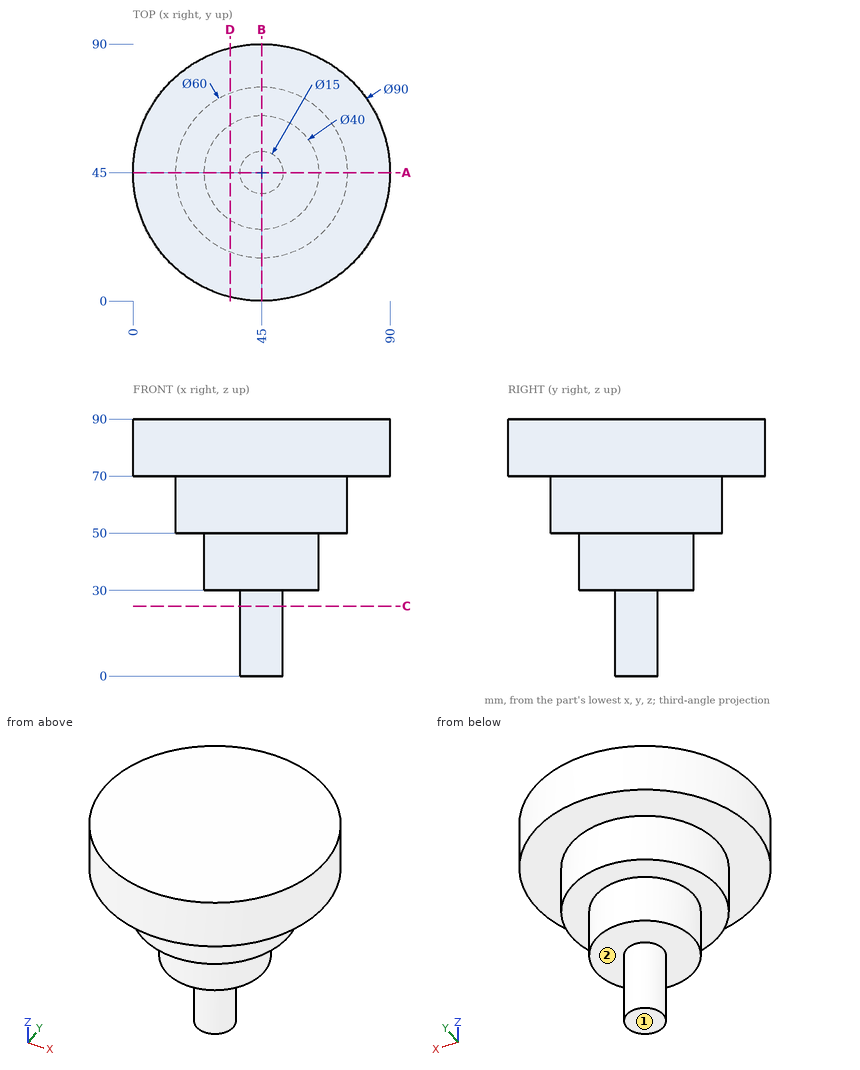
Can you work these out from the drawing? Everything is in mm from the part's minimum corner. A direction names the side the tool comes from. Round coordinates to 2 decimals unless told otherwise and drop trailing zeros. Loops run counter-clockwise (first coordinate to the right, second up) from the corner with the lowest first, then second, coordinate; pieces in that order, holes last. Notation, with made-up numbers: (-22, 10) -> (-4, 10) arc R23 cw to (-4, 23) -> close; hole circle Ø5 at (50.25, 34). An arc over 180 degrees is marked (long way). Answer in a Markdown table with one row per item.
Item 1: Suppose I cut it at D-D, the plane x = 34. List the corners of the cut face in (y, z) for me, plus the area to 3 significant figures.
Answer block:
| item | result |
|---|---|
| outline | (1.37, 70) -> (17.09, 70) -> (17.09, 50) -> (28.3, 50) -> (28.3, 30) -> (61.7, 30) -> (61.7, 50) -> (72.91, 50) -> (72.91, 70) -> (88.63, 70) -> (88.63, 90) -> (1.37, 90) -> close |
| area | 3,530 mm² |
Item 2: Suppose I cut it at A-A, the plane y = 45. List the corners of the cut face in (x, z) for me.
Answer block:
| item | result |
|---|---|
| outline | (0, 70) -> (15, 70) -> (15, 50) -> (25, 50) -> (25, 30) -> (37.5, 30) -> (37.5, 0) -> (52.5, 0) -> (52.5, 30) -> (65, 30) -> (65, 50) -> (75, 50) -> (75, 70) -> (90, 70) -> (90, 90) -> (0, 90) -> close |
Item 3: Suppose I cut it at C-C, the plane z = 24.5. List the corners of the cut face in (x, y) for me.
Answer block:
| item | result |
|---|---|
| outline | circle Ø15 at (45, 45) |
Item 4: If I drill on probe 1 along Z at (x, y) = (32, 46.5); probe 2 along X at (y, z) = (46.5, 85) (3 decimals); probe 3 along X at (y, z) = (45, 69), over which ranges is the centre line in solid material (lowest first)?
Answer block:
| item | result |
|---|---|
| probe 1 | 30 to 90 |
| probe 2 | 0.025 to 89.975 |
| probe 3 | 15 to 75 |
Item 5: Will these pins go through, and if not, where does the flat tip stop? P1, Ø3, axis at x = 41, z = 66, coming from the +Y side; P2, Ø12, axis at y = 29, z = 54, coming from the +X side; P3, Ø1.5, axis at y = 76.5, z = 57, coming from the -X side; P4, Ø1, axis at x = 17, y = 45.5, coming from the -Z side.
Answer block:
| item | result |
|---|---|
| P1 | y = 74.9 |
| P2 | x = 73.28 |
| P3 | through |
| P4 | z = 50 |
Item 6: On a 3-axis mill with a long thin cutter (end or side, diameter ignored), from which of +Z, -Z, +X, -X, +Y, -Y can I reach the whole of each face in a straight line? I mean the marked faces 1 and 2. Say none if no direction works.
Answer block:
| item | result |
|---|---|
| face 1 | -Z, +X, -X, +Y, -Y |
| face 2 | -Z |
